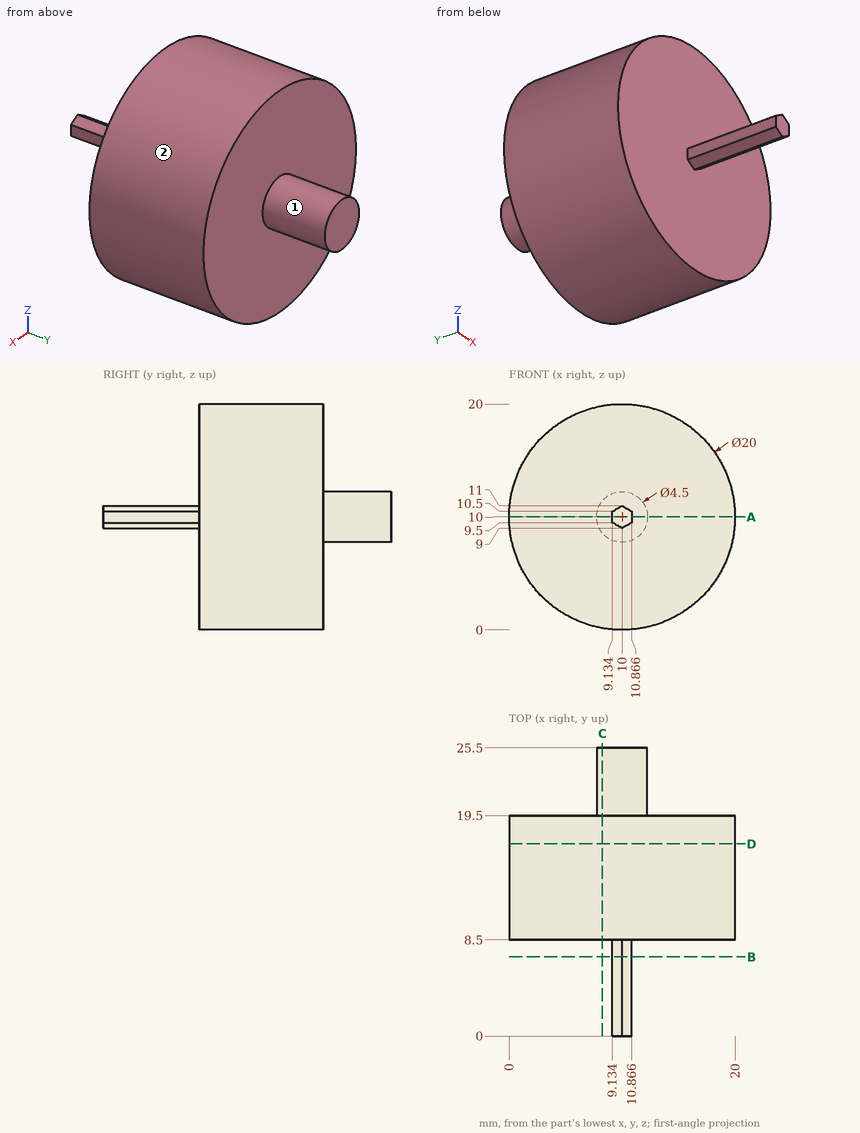
Study the drawing (mm; zero at the part's minimum x, y, z) and answer. A direction names the side the tool comes from. Coordinates: 2 decimals unless noted, no trailing zeros. Write each loop counter-clockwise with the first axis right and the second up, starting at its lowest first coordinate (ties: lowest second). Pieces come first, ordered by that corner, then holes. Notation, with made-up numbers: (-4, -18) - (3, -18) arc R22 ccw to (3, 0) - close; hole circle Ø9 at (76.25, 3.5). An arc over 180 degrees is marked (long way). Answer as a JSON object with one key per item and string values. Group by question number.
1. A cutting plane is placed at C-C (x = 8.25). Determine the outline of the cut face in (y, z).
2. A cutting plane is placed at A-A (z = 10). Determine the outline of the cut face in (x, y), plus the area to 3 significant figures.
3. Each of these flat-tipped pins is pushed along its axis until it touches: P1, Ø4, axis at x = 16, y = 14, coming from the +Z side; P2, Ø2, axis at y = 14, z = 15.5, coming from the +X side; P3, Ø4, axis at x = 7, z = 9, coming from the -Y side. Where does it stop, or does it pass through?
4. Which of the six approach directions +Z, -Z, +X, -X, +Y, -Y give full straight-line access (tool end or side, diameter ignored) to the marked faces 1 and 2?
5. A cutting plane is placed at B-B (y = 7). Determine the outline of the cut face in (x, z).
6. Consider L1, parallel to Y at x = 2.25, z = 4.5; L2, parallel to Y at x = 8.5, z = 10.5; L3, parallel to X at y = 9, z = 7.75. Determine where each line is inside the solid, lowest interval first. Write a range as [from, to].
7. A cutting plane is placed at D-D (y = 17). Determine the outline of the cut face in (x, z).
Worked out:
{
 "1": {"outline": "(8.5, 0.15) - (19.5, 0.15) - (19.5, 8.59) - (25.5, 8.59) - (25.5, 11.41) - (19.5, 11.41) - (19.5, 19.85) - (8.5, 19.85) - close"},
 "2": {"outline": "(0, 8.5) - (9.13, 8.5) - (9.13, 0) - (10.87, 0) - (10.87, 8.5) - (20, 8.5) - (20, 19.5) - (12.25, 19.5) - (12.25, 25.5) - (7.75, 25.5) - (7.75, 19.5) - (0, 19.5) - close", "area": "262 mm²"},
 "3": {"P1": "stops at z = 19.17", "P2": "stops at x = 18.93", "P3": "stops at y = 8.5"},
 "4": {"face 1": "+Y", "face 2": "+Y, -Y"},
 "5": {"outline": "(9.13, 9.5) - (10, 9) - (10.87, 9.5) - (10.87, 10.5) - (10, 11) - (9.13, 10.5) - close"},
 "6": {"L1": "y = [8.5, 19.5]", "L2": "y = [8.5, 25.5]", "L3": "x = [0.26, 19.74]"},
 "7": {"outline": "circle Ø20 at (10, 10)"}
}
